Geometry check sheet. Reference: the model listing, model coordinates, mm. Face numbers are marked on the shaded views. A direction names the side the tool comes from. Give positions to 0.01 mm unless a question says otherwise; leave off trailing zeros. Write each loop counter-clockwise with the first axis right and the second up, starting at its lowest first coordinate (ties: lowest second). Pieces come first, ordered by that corner, then holes. Notation, with made-up numbers: M -39.75,82 L 15.25,82 A32 cw 15.25,109 Z; hole C 22,60 d4. An arc over 180 degrees is marked long. Write each question's results on one line, items separated by ' | '.
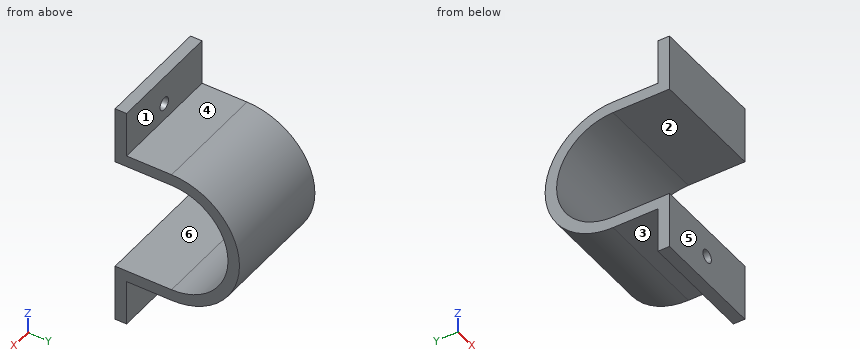
Autodesk Inventor part; units mm, degrees
ref_plane "YZ Plane" through (0, 0, 0) normal (1, 0, 0) x (0, 1, 0)
ref_plane "XZ Plane" through (0, 0, 0) normal (0, 1, 0) x (-1, 0, 0)
ref_plane "XY Plane" through (0, 0, 0) normal (0, 0, 1) x (1, 0, 0)
sketch "Sketch1" plane through (0, 0, 0) normal (1, 0, 0) x (0, 1, 0)
  arc A0 (0, -12.5) -> (0, 12.5) centre (0, 0) ccw
  line L0 (-12.5, -25.2) -> (-9.96, -25.2)
  line L1 (-9.96, -25.2) -> (-9.96, -15.04)
  line L2 (-12.5064, 25.2) -> (-9.9664, 25.2)
  line L3 (-12.5064, 25.2) -> (-12.5064, 12.5)
  line L4 (-12.5, -12.5) -> (-12.5, -25.2)
  line L5 (-9.9664, 15.04) -> (-9.9664, 25.2)
  arc A1 (0, -15.04) -> (0, 15.04) centre (0, 0) ccw
  line L6 (0, 15.04) -> (-9.9664, 15.04)
  line L7 (0, 12.5) -> (-12.5064, 12.5)
  line L8 (0, -12.5) -> (-12.5, -12.5)
  line L9 (0, -15.04) -> (-9.96, -15.04)
  point P0 (-4.98, -15)
  dimension "d0" = 25
  dimension "d9" = 12.7
  dimension "d10" = 12.7
  dimension "d11" = 2.54
  dimension "d12" = 2.54
  dimension "d15" = 2.54
  dimension "d17" = 0.0064
  dimension "d23" = 0
  dimension "d24" = 0
  dimension "d25" = 0
  dimension "d26" = 0
  dimension "d27" = 0.04
  dimension "d28" = 4.98
extrude "Extrusion1" add sketch "Sketch1" along normal blind 25.4
sketch "Sketch2" plane through (0, -12.5, -25.2) normal (0, -1, 0) x (1, 0, 0)
  circle A0 centre (12.7, 44.05) radius 1.4224
  circle A1 centre (12.7, 6.35) radius 1.4224
  line L0 (0, 50.4) -> (25.4, 50.4)
  line L1 (25.4, 50.4) -> (25.4, 37.7)
  line L2 (0, 0) -> (25.4, 0)
  point P0 (0, 25.2)
  dimension "d31" = 2.8448
  dimension "d32" = 6.35
  dimension "d33" = 12.7
  dimension "d34" = 0
  dimension "d35" = 6.35
  dimension "d36" = 2.8448
extrude "Extrusion2" cut sketch "Sketch2" against normal blind 25.4
properties part number "Motor mount"
Q1. Release check for a two-part mould opening along Z. For the marked faces 4, 5 and 6 record: released by +Z, released by -Z, zero draft, split by the parting line, or undercut.
Answer key:
face 4: released by +Z | face 5: zero draft | face 6: undercut
Q2. Depth check by flat-ended pin: P1, Ø12, axis at x = 10.5, y = 11, coming from the +Z side; P2, Ø5, axis at x = 21, y = -4.5, coming from the +Z side; P3, Ø8, axis at x = 3, z = -0.5, coming from the -Y side. Enter the tip coordinate at first touch or a pass-through.
Answer key:
P1: stops at z = 14.18 | P2: stops at z = 15.04 | P3: stops at y = 11.66
Q3. Section check C-C (y = 4.75). Enter the section's corners in (x, z).
Answer key:
outline: M 0,-14.27 L 25.4,-14.27 L 25.4,-11.56 L 0,-11.56 Z; M 0,11.56 L 25.4,11.56 L 25.4,14.27 L 0,14.27 Z
Q4. Section check B-B (z = -18.85). Enter the section's corners in (x, y).
Answer key:
outline: M 0,-12.5 L 11.28,-12.5 L 11.28,-9.96 L 0,-9.96 Z; M 14.12,-12.5 L 25.4,-12.5 L 25.4,-9.96 L 14.12,-9.96 Z
Q5. Section check D-D (x = 21.5). Enter the section's corners in (y, z), then the cut area to 3 significant figures.
Answer key:
outline: M -12.51,12.5 L 0,12.5 A12.5 cw 0,-12.5 L -12.5,-12.5 L -12.5,-25.2 L -9.96,-25.2 L -9.96,-15.04 L 0,-15.04 A15.04 ccw 0,15.04 L -9.97,15.04 L -9.97,25.2 L -12.51,25.2 Z | area: 225 mm2
Q6. Material ranges on probe 1 along Z at (x, y) = (12.7, -10.9); probe 2 along Z at (x, y) = (19, -2.75); probe 3 along Z at (x, y) = (8.75, 9.5), recorded low to high. Write a range as [from, to].
Answer key:
probe 1: z = [-25.2, -20.27], [-17.43, -12.5], [12.5, 17.43], [20.27, 25.2] | probe 2: z = [-15.04, -12.5], [12.5, 15.04] | probe 3: z = [-11.66, -8.12], [8.12, 11.66]
Q7. Access from +Z, -Z, +X, -X, +Y, -Y to the whole of each face (thin tool, end or side, straight path). Record for the marked faces 1, 2 and 3.
Answer key:
face 1: +Z, +X, -X, +Y | face 2: +X, -X, -Y | face 3: -Z, +X, -X, +Y
Q8. Section check A-A (x = 12.7). Enter the section's corners in (y, z), then the cut area to 3 significant figures.
Answer key:
outline: M -12.51,12.5 L 0,12.5 A12.5 cw 0,-12.5 L -12.5,-12.5 L -12.5,-17.43 L -9.96,-17.43 L -9.96,-15.04 L 0,-15.04 A15.04 ccw 0,15.04 L -9.97,15.04 L -9.97,17.43 L -12.5,17.43 L -12.5,20.27 L -9.97,20.27 L -9.97,25.2 L -12.51,25.2 Z; M -12.5,-25.2 L -9.96,-25.2 L -9.96,-20.27 L -12.5,-20.27 Z | area: 211 mm2
